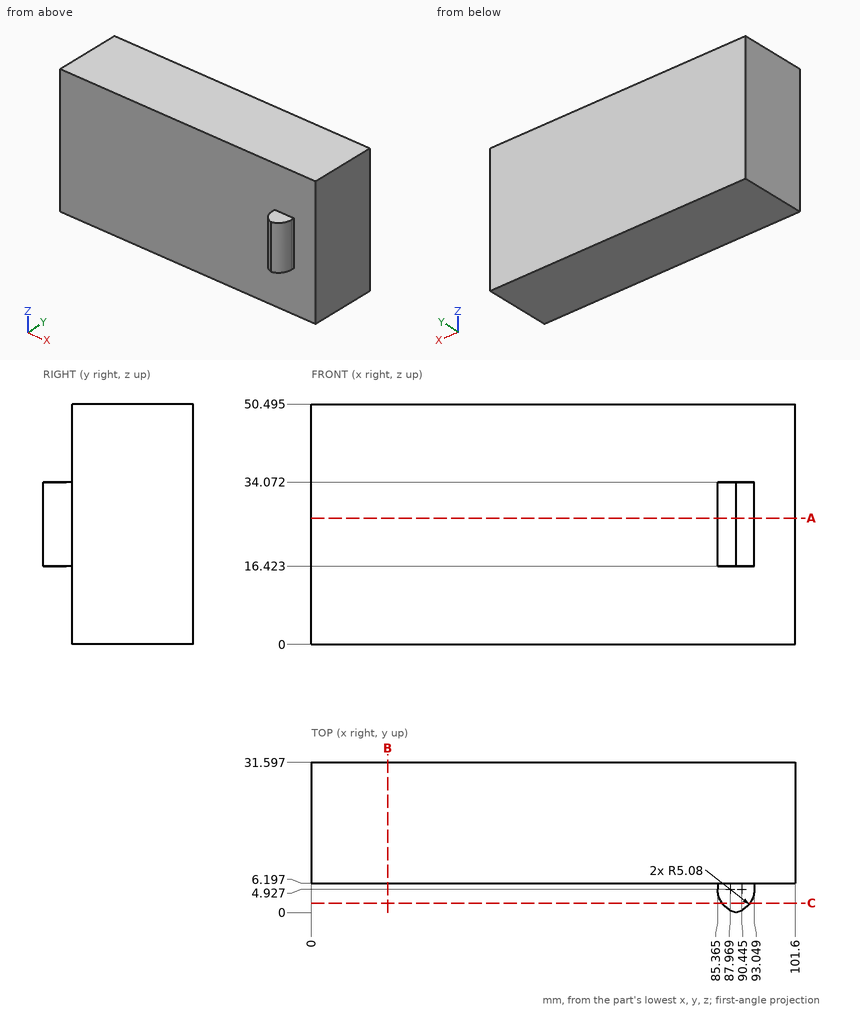
Answer from the drawing. Dimensions are ordinates in mm from the lowest x, y and z of the part. Give positions to 0.01 mm unless a question says otherwise; leave off trailing zeros. Write each loop counter-clockwise with the first axis right and the second up, starting at its lowest first coordinate (ties: lowest second). Pieces come first, ordered by that corner, then holes.
1) Given P1, Ø1.9, axis at x = 90.5, y = 2, coming from the -Z side; P2, Ø25, axis at x = 44, z = 33, coming from the -Y side; P3, Ø3, axis at x = 11, y = 27.5, coming from the -Z side; P4, Ø1, axis at y = 5.5, z = 22, coming from the -X side (3 decimals), each flat-ended and moving along its own axis, determine where each tip first touches the part or whether it passes through.
2) Section A-A (z = 26.5) is taken. Write down the section's boundary in (x, y) (1 decimal).
3) Section B-B (x = 16) is taken. Write down the section's boundary in (y, z) (1 decimal), and give its area (3 significant figures).
4) Section C-C (y = 2) is taken. Write down the section's boundary in (x, z), and give its area (3 significant figures).
5) Find the intervals of material crossed by L1, parallel to Y at x = 63, z = 48.5, in increasing order.
Response:
1. P1: stops at z = 16.42
1. P2: stops at y = 6.2
1. P3: stops at z = 0
1. P4: stops at x = 85.365
2. outline: (0, 6.2) - (85.4, 6.2) - (85.4, 4.9) arc R5.1 ccw to (89.2, 0) arc R5.1 ccw to (93, 4.9) - (93, 6.2) - (101.6, 6.2) - (101.6, 31.6) - (0, 31.6) - close
3. outline: (6.2, 0) - (31.6, 0) - (31.6, 50.5) - (6.2, 50.5) - close
3. area: 1,280 mm2
4. outline: (86.29, 16.42) - (92.12, 16.42) - (92.12, 34.07) - (86.29, 34.07) - close
4. area: 103 mm2
5. L1: y = 6.2 to 31.6
